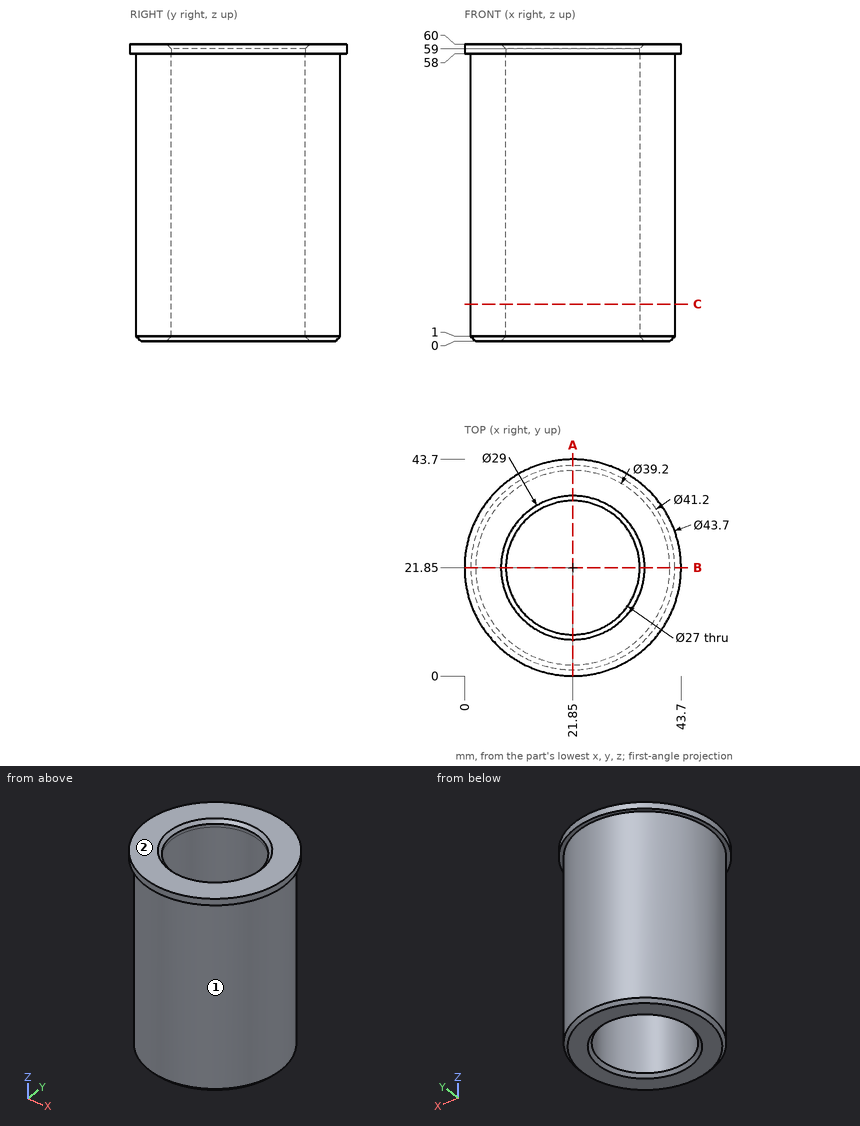
Answer from the drawing. Dimensions are ordinates in mm from the lowest x, y and z of the part. A direction names the side the tool comes from. Round coordinates to 2 decimals unless told otherwise and drop trailing zeros. Loops run counter-clockwise (first coordinate to the right, second up) from the corner with the lowest first, then second, coordinate; pieces in that order, holes last.
(1) The part is cut by section C-C, the plane z = 7.5. Give the vertices of the cut face in (x, y).
Computed values:
outline: circle Ø41.2 at (21.85, 21.85); hole circle Ø27 at (21.85, 21.85)
(2) For the marked faces 1 and 2, determine the directions among +Z, -Z, +X, -X, +Y, -Y from which every point of the face is accessible in a straight line to the end or side of a thin tool.
Computed values:
face 1: -Z
face 2: +Z, +X, -X, +Y, -Y
(3) Each of these flat-tipped pins is pushed along its axis until it touches: P1, Ø8, axis at x = 19, z = 16, coming from the -Y side; P2, Ø1, axis at x = 22, z = 45, coming from the +Y side; P3, Ø1.5, axis at x = 35.5, y = 5.5, coming from the -Z side. Where does it stop, or does it pass through?
Computed values:
P1: stops at y = 1.25
P2: stops at y = 42.45
P3: stops at z = 0.95
(4) Find the intervals of material crossed by L1, parallel to Y at x = 21.85, z = 58.2; L2, parallel to X at y = 13, z = 44.5; L3, parallel to Y at x = 33.5, z = 31.5, in increasing order.
Computed values:
L1: y = 0 to 8.35, 35.35 to 43.7
L2: x = 3.25 to 11.66, 32.04 to 40.45
L3: y = 4.86 to 15.03, 28.67 to 38.84
(5) The part is cut by section A-A, the plane x = 21.85. Give the vertices of the cut face in (y, z).
Computed values:
outline: (0, 58) - (1.25, 58) - (1.25, 1) - (2.25, 0) - (7.35, 0) - (8.35, 1) - (8.35, 59) - (7.35, 60) - (0, 60) - close; (35.35, 1) - (36.35, 0) - (41.45, 0) - (42.45, 1) - (42.45, 58) - (43.7, 58) - (43.7, 60) - (36.35, 60) - (35.35, 59) - close
